Verification items for the finished model (mm, model axes). Face numbers are marked on the shaded views. A direction names the side the tool comes from. Round coordinates to 2 decimals unless told otherwise and drop trailing zeros. Order: outer loops, then holes, each group sorted by start corner. A loop starts at its lowest first (then second) coordinate and runs counter-clockwise, first axis right, second up. Notation, with made-up numbers: (42.5, -37) -> (62.5, -37) arc R22 cw to (62.5, -1) -> close; hole circle Ø1 at (-17.75, 71). An arc over 180 degrees is marked (long way). Write item = value, one per line. Start each with the question number.
from build123d import *

# Parameters (mm, degrees)
F0_W     = 15.97
F0_H     = 15.97
F1_DEPTH = 1.5
F2_DEPTH = 6
F3_DEPTH = 14
F4_R     = 0.5
F5_DEPTH = 25
F7_D     = 3


# Not quite as in the source:
# - after a boolean that leaves OpenCascade's solid faulty, fix() repairs it


with BuildPart() as f1:
    # F0 (on Top) → F1 (new body)
    with BuildSketch(Plane.XY):
        Polygon((11.463976, 2.379747), (11.359373, 2.838321), (11.236939, 3.290208), (11.097035, 3.735011), (10.940019, 4.172325), (10.766249, 4.60174), (10.576084, 5.022839), (10.369884, 5.435203), (10.148011, 5.838407), (9.910829, 6.232024), (9.658704, 6.615624), (9.392003, 6.988776), (9.111097, 7.351047), (8.816357, 7.702006), (8.508156, 8.04122), (8.186868, 8.368258), (7.852869, 8.68269), (7.506532, 8.98409), (7.148231, 9.272031), (6.778339, 9.546091), (6.397225, 9.805849), (6.005257, 10.050886), (5.602798, 10.280786), (5.190206, 10.495134), (4.767834, 10.693518), (4.336029, 10.875525), (3.895133, 11.040743), (3.851403, 11.055137), (-0.000321, 8.82993), (-3.850041, 11.056837), (-3.888073, 11.04433), (-4.324324, 10.88112), (-4.752184, 10.701192), (-5.171268, 10.504934), (-5.581182, 10.292736), (-5.98153, 10.06499), (-6.371909, 9.822089), (-6.751914, 9.564429), (-7.121137, 9.292409), (-7.47917, 9.00643), (-7.825602, 8.706896), (-8.160021, 8.394212), (-8.482018, 8.068787), (-8.791184, 7.73103), (-9.087111, 7.38135), (-9.369393, 7.020158), (-9.637626, 6.647865), (-9.89141, 6.26488), (-10.130347, 5.871608), (-10.354039, 5.468455), (-10.562095, 5.055822), (-10.754123, 4.634103), (-10.929732, 4.203692), (-11.088533, 3.764972), (-11.230138, 3.318323), (-11.354158, 2.864116), (-11.4602, 2.402716), (-11.54787, 1.934479), (-11.616771, 1.459754), (-11.666499, 0.978883), (-11.696643, 0.4922), (-11.706789, -8e-05), (-11.696889, -0.484214), (-11.667434, -0.963844), (-11.618789, -1.43855), (-11.551313, -1.907948), (-11.465359, -2.371647), (-11.36128, -2.829248), (-11.239422, -3.280348), (-11.100133, -3.724535), (-10.943759, -4.161393), (-10.770647, -4.590499), (-10.581144, -5.011426), (-10.375599, -5.423743), (-10.154362, -5.827016), (-9.917785, -6.220806), (-9.666223, -6.604675), (-9.400031, -6.978182), (-9.119567, -7.340886), (-8.825191, -7.692347), (-8.517263, -8.032124), (-8.196144, -8.359779), (-7.862195, -8.674874), (-7.515776, -8.976975), (-7.157247, -9.265648), (-6.786965, -9.540464), (-6.405285, -9.800995), (-6.012557, -10.046813), (-5.609128, -10.277496), (-5.195341, -10.492621), (-4.771529, -10.691767), (-4.338024, -10.874511), (-3.895147, -11.040433), (-3.849233, -11.055538), (0.000108, -8.829807), (3.850042, -11.056838), (3.888074, -11.04433), (4.324324, -10.881121), (4.752185, -10.701192), (5.171269, -10.504935), (5.581183, -10.292737), (5.98153, -10.064991), (6.371909, -9.822089), (6.751914, -9.56443), (7.121138, -9.29241), (7.479171, -9.006431), (7.825602, -8.706896), (8.160022, -8.394213), (8.482019, -8.068788), (8.791185, -7.73103), (9.087111, -7.38135), (9.369393, -7.020159), (9.637626, -6.647866), (9.891411, -6.26488), (10.130347, -5.871609), (10.35404, -5.468456), (10.562096, -5.055822), (10.754123, -4.634104), (10.929732, -4.203692), (11.088534, -3.764973), (11.230139, -3.318324), (11.354158, -2.864117), (11.4602, -2.402716), (11.547871, -1.934479), (11.616772, -1.459754), (11.666499, -0.978883), (11.696644, -0.492201), (11.706789, 5.7e-05), (11.696823, 0.486311), (11.667183, 0.967786), (11.618247, 1.444099), (11.550389, 1.914878), align=None)
        Rectangle(F0_W, F0_H, mode=Mode.SUBTRACT)
    extrude(amount=F1_DEPTH)

    # F0 (on Top) → F2 (join)
    with BuildSketch(Plane.XY):
        Rectangle(F0_W, F0_H)
        with BuildLine():
            ThreePointArc((-5.5, 0), (-3.8890872965, 3.8890872965), (0, 5.5))
            ThreePointArc((0, 5.5), (3.8890872965, 3.8890872965), (5.5, 0))
            ThreePointArc((5.5, 0), (3.8890872965, -3.8890872965), (0, -5.5))
            ThreePointArc((0, -5.5), (-3.8890872965, -3.8890872965), (-5.5, 0))
        make_face(mode=Mode.SUBTRACT)
    extrude(amount=F2_DEPTH)

    # F0 (on Top) → F3 (join)
    with BuildSketch(Plane.XY):
        with BuildLine():
            ThreePointArc((5.5, 0), (3.8890872965, 3.8890872965), (0, 5.5))
            ThreePointArc((0, 5.5), (-3.8890872965, 3.8890872965), (-5.5, 0))
            ThreePointArc((-5.5, 0), (-3.8890872965, -3.8890872965), (0, -5.5))
            ThreePointArc((0, -5.5), (3.8890872965, -3.8890872965), (5.5, 0))
        make_face()
        with BuildLine():
            ThreePointArc((-3, 0), (-2.1213203436, 2.1213203436), (0, 3))
            ThreePointArc((0, 3), (2.1213203436, 2.1213203436), (3, 0))
            ThreePointArc((3, 0), (2.1213203436, -2.1213203436), (0, -3))
            ThreePointArc((0, -3), (-2.1213203436, -2.1213203436), (-3, 0))
        make_face(mode=Mode.SUBTRACT)
    extrude(amount=F3_DEPTH)

    # F4
    f4_edges = [f1.edges().sort_by_distance(p)[0] for p in [
        (-7.985, 0, 6),
        (0, -7.985, 6),
        (7.985, 0, 6),
        (0, 7.985, 6),
    ]]
    fillet(f4_edges, radius=F4_R)

    # F0 (on Top) → F5 (join)
    with BuildSketch(Plane.XY):
        with BuildLine():
            ThreePointArc((5.5, 0), (3.8890872965, 3.8890872965), (0, 5.5))
            ThreePointArc((0, 5.5), (-3.8890872965, 3.8890872965), (-5.5, 0))
            ThreePointArc((-5.5, 0), (-3.8890872965, -3.8890872965), (0, -5.5))
            ThreePointArc((0, -5.5), (3.8890872965, -3.8890872965), (5.5, 0))
        make_face()
        with BuildLine():
            ThreePointArc((-3, 0), (-2.1213203436, 2.1213203436), (0, 3))
            ThreePointArc((0, 3), (2.1213203436, 2.1213203436), (3, 0))
            ThreePointArc((3, 0), (2.1213203436, -2.1213203436), (0, -3))
            ThreePointArc((0, -3), (-2.1213203436, -2.1213203436), (-3, 0))
        make_face(mode=Mode.SUBTRACT)
    extrude(amount=F5_DEPTH)

    # F7 (through all)
    with Locations(Plane(origin=(-7.985, 0, 0), x_dir=(0, -1, 0), z_dir=(-1, 0, 0))):
        with Locations((0, 3.5)):
            Hole(F7_D / 2)

    add(f1.part.fix(), mode=Mode.REPLACE)


solid = f1.part
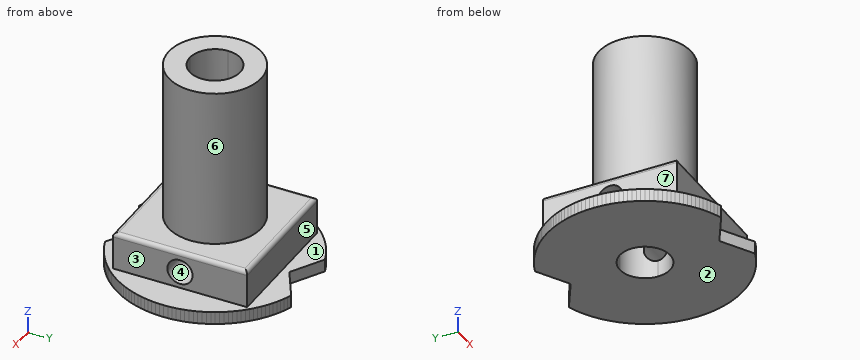
(1) Cross-section at B-B (x = 2.25). Enter the section's corners in (y, z) (3 decimals), and give its area (3 significant figures).
(2) Draft check along Z on the marked faces 1, 2, 3 and 4. Enter one of: +Z half, -Z half, draft (parallel to the pull), parting line (faces both ways), or undercut.
(3) Cross-section at A-A (z = 3.5). Enter the section's corners in (x, y) (3 decimals).
(4) Cross-section at D-D (x = -3.5). Enter the section's corners in (y, z) (3 decimals).
(5) Scan lines: line 1 along Z through (x, y) = (-5.2, 0); line 2 along Y through (x, z) = (-6.3, 3.5) (3 decimals); line 3 along X through (y, z) = (1.5, 8.75). Record each from-to range of solid material in increasing order. Write a range as from..to.
(6) Depth check by flat-ended pin: pin 1 (8 mm diameter, centred on y = 6, z = 8, fed in from +X) (3 decimals); pin 2 (2.5 mm diameter, centred on y = 0, z = 3.5, fed in from -X); pin 3 (1.2 mm diameter, centred on x = -0.5, z = 4, fed in from -Y) (3 decimals); pin 4 (2 mm diameter, centred on x = 0, z = 3.5, fed in from +Y) (3 decimals). Enter the tip coordinate at first touch or a pass-through.
(7) Set-up check for the marked faces 5, 6 and 7: record each of +Z, -Z, +X, -X, +Y, -Y from which the full face is reachable in a straight line by a thin tool's end or side.
(8) Cross-section at C-C (z = 12.5). Enter the section's corners in (x, y).
Outcome:
q1.outline = (-10.131, 0) -> (-1.984, 0) -> (-1.984, 25) -> (-5.019, 25) -> (-5.019, 6) -> (-7.485, 6) arc R0.5 ccw to (-7.985, 5.5) -> (-7.985, 1.5) -> (-10.131, 1.5) -> close; (1.984, 0) -> (10.13, 0) -> (10.13, 1.5) -> (7.985, 1.5) -> (7.985, 5.5) arc R0.5 ccw to (7.485, 6) -> (5.019, 6) -> (5.019, 25) -> (1.984, 25) -> close
q1.area = 194 mm^2
q2.face_1 = +Z half
q2.face_2 = -Z half
q2.face_3 = draft
q2.face_4 = undercut
q3.outline = (-7.985, -7.985) -> (7.985, -7.985) -> (7.985, -1.5) -> (2.598, -1.5) arc R3 cw to (-2.598, -1.5) -> (-7.985, -1.5) -> close; (-7.985, 1.5) -> (-2.598, 1.5) arc R3 cw to (2.598, 1.5) -> (7.985, 1.5) -> (7.985, 7.985) -> (-7.985, 7.985) -> close
q4.outline = (-10.854, 0) -> (10.854, 0) -> (10.854, 1.5) -> (7.985, 1.5) -> (7.985, 5.5) arc R0.5 ccw to (7.485, 6) -> (4.243, 6) -> (4.243, 25) -> (-4.243, 25) -> (-4.243, 6) -> (-7.485, 6) arc R0.5 ccw to (-7.985, 5.5) -> (-7.985, 1.5) -> (-10.854, 1.5) -> close; hole circle Ø3 at (0, 3.5)
q5.line_1 = 0..2, 5..25
q5.line_2 = -7.985..-1.5, 1.5..7.985
q5.line_3 = -5.29..-2.6, 2.6..5.29
q6.pin_1 = 7.985
q6.pin_2 = through
q6.pin_3 = -7.985
q6.pin_4 = 7.985
q7.face_5 = +Z, +X, -X, +Y
q7.face_6 = +Z
q7.face_7 = +Z, -X, +Y, -Y
q8.outline = circle Ø11 at (0, 0); hole circle Ø6 at (0, 0)
